Can you work these out from the model? Positions are in its coordinate system, mm. Give positions to 0.01 mm unless a question says otherwise; leave off trailing zeros. Order: outer loops, then holes, each group sorted by start corner. A loop starts at its lowest first (then second) coordinate and runs counter-clockwise, first axis right, second up. Notation, with made-up numbers: (26.5, 19) - (84.5, 19) arc R24 cw to (84.5, 31) - close; hole circle Ø9 at (12, 32.25). An arc over 180 degrees is marked (long way). Answer as a JSON object with one key per item and string values.
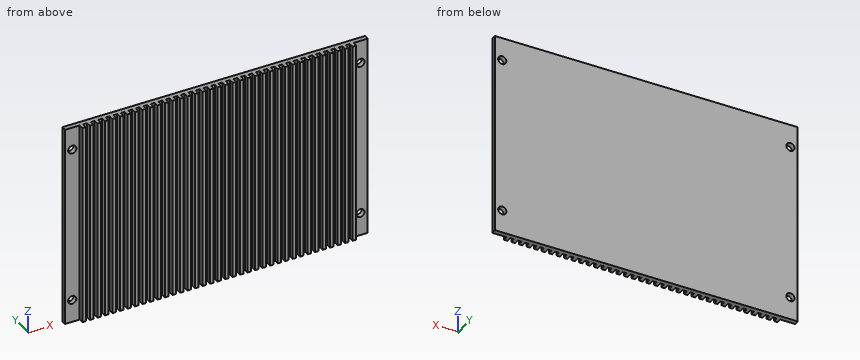
```python
from build123d import *

# Parameters (mm, degrees)
SKETCH1_W               = 125
SKETCH1_H               = 84
BOSS_EXTRUDE1_DEPTH     = 2
M3_CLEARANCE_HOLE1_D    = 3.4
MIRROR2_COPY_1_D        = 3.4
SKETCH4_W               = 1.5
SKETCH4_H               = 84
BOSS_EXTRUDE2_DEPTH     = 2
FILL_START              = -42
FILL_PATTERN2_OUTLINE_W = 1.5
FILL_PATTERN2_OUTLINE_H = 2
FILL_PATTERN2_DEPTH     = 84


# Read off the part's stored shape, not the designer's step: Fill Pattern2
with BuildPart() as part:
    # Sketch1 → Boss-Extrude1 (new body)
    with BuildSketch(Plane(origin=(0, 0, 0), x_dir=(1, 0, 0), z_dir=(0, 1, 0))):
        Rectangle(SKETCH1_W, SKETCH1_H)
    extrude(amount=BOSS_EXTRUDE1_DEPTH)

    # M3 Clearance Hole1 (through all)
    with Locations(Plane(origin=(0, 2, 0), x_dir=(1, 0, 0), z_dir=(0, 1, 0))):
        with Locations((-59.5, 32.5)):
            m3_clearance_hole1 = Hole(M3_CLEARANCE_HOLE1_D / 2)

    # Mirror1: M3 Clearance Hole1 across plane
    add(m3_clearance_hole1.mirror(Plane(origin=(0, 0, 0), x_dir=(0, 0, 1), z_dir=(1, 0, 0))), mode=Mode.SUBTRACT)

    # Mirror2: M3 Clearance Hole1 across plane
    add(m3_clearance_hole1.mirror(Plane.XY), mode=Mode.SUBTRACT)

    # Mirror2 copy 1 (through all)
    with Locations(Plane(origin=(0, 2, 0), x_dir=(-1, 0, 0), z_dir=(0, 1, 0))):
        with Locations((-59.5, 32.5)):
            Hole(MIRROR2_COPY_1_D / 2)

    # Sketch4 → Boss-Extrude2 (add)
    with BuildSketch(Plane(origin=(0, 0, 0), x_dir=(1, 0, 0), z_dir=(0, 1, 0))):
        with Locations((-55.7, 0)):
            Rectangle(SKETCH4_W, SKETCH4_H)
    extrude(amount=-BOSS_EXTRUDE2_DEPTH)

    # Fill Pattern2 outline → Fill Pattern2 (add)
    with BuildSketch(Plane.XY.offset(FILL_START)):
        with Locations((55.9, -1)):
            Rectangle(FILL_PATTERN2_OUTLINE_W, FILL_PATTERN2_OUTLINE_H)
        with Locations((52.8, -1)):
            Rectangle(FILL_PATTERN2_OUTLINE_W, FILL_PATTERN2_OUTLINE_H)
        with Locations((49.7, -1)):
            Rectangle(FILL_PATTERN2_OUTLINE_W, FILL_PATTERN2_OUTLINE_H)
        with Locations((46.6, -1)):
            Rectangle(FILL_PATTERN2_OUTLINE_W, FILL_PATTERN2_OUTLINE_H)
        with Locations((43.5, -1)):
            Rectangle(FILL_PATTERN2_OUTLINE_W, FILL_PATTERN2_OUTLINE_H)
        with Locations((40.4, -1)):
            Rectangle(FILL_PATTERN2_OUTLINE_W, FILL_PATTERN2_OUTLINE_H)
        with Locations((37.3, -1)):
            Rectangle(FILL_PATTERN2_OUTLINE_W, FILL_PATTERN2_OUTLINE_H)
        with Locations((34.2, -1)):
            Rectangle(FILL_PATTERN2_OUTLINE_W, FILL_PATTERN2_OUTLINE_H)
        with Locations((31.1, -1)):
            Rectangle(FILL_PATTERN2_OUTLINE_W, FILL_PATTERN2_OUTLINE_H)
        with Locations((28, -1)):
            Rectangle(FILL_PATTERN2_OUTLINE_W, FILL_PATTERN2_OUTLINE_H)
        with Locations((24.9, -1)):
            Rectangle(FILL_PATTERN2_OUTLINE_W, FILL_PATTERN2_OUTLINE_H)
        with Locations((21.8, -1)):
            Rectangle(FILL_PATTERN2_OUTLINE_W, FILL_PATTERN2_OUTLINE_H)
        with Locations((18.7, -1)):
            Rectangle(FILL_PATTERN2_OUTLINE_W, FILL_PATTERN2_OUTLINE_H)
        with Locations((15.6, -1)):
            Rectangle(FILL_PATTERN2_OUTLINE_W, FILL_PATTERN2_OUTLINE_H)
        with Locations((12.5, -1)):
            Rectangle(FILL_PATTERN2_OUTLINE_W, FILL_PATTERN2_OUTLINE_H)
        with Locations((9.4, -1)):
            Rectangle(FILL_PATTERN2_OUTLINE_W, FILL_PATTERN2_OUTLINE_H)
        with Locations((6.3, -1)):
            Rectangle(FILL_PATTERN2_OUTLINE_W, FILL_PATTERN2_OUTLINE_H)
        with Locations((3.2, -1)):
            Rectangle(FILL_PATTERN2_OUTLINE_W, FILL_PATTERN2_OUTLINE_H)
        with Locations((0.1, -1)):
            Rectangle(FILL_PATTERN2_OUTLINE_W, FILL_PATTERN2_OUTLINE_H)
        with Locations((-3, -1)):
            Rectangle(FILL_PATTERN2_OUTLINE_W, FILL_PATTERN2_OUTLINE_H)
        with Locations((-6.1, -1)):
            Rectangle(FILL_PATTERN2_OUTLINE_W, FILL_PATTERN2_OUTLINE_H)
        with Locations((-9.2, -1)):
            Rectangle(FILL_PATTERN2_OUTLINE_W, FILL_PATTERN2_OUTLINE_H)
        with Locations((-12.3, -1)):
            Rectangle(FILL_PATTERN2_OUTLINE_W, FILL_PATTERN2_OUTLINE_H)
        with Locations((-15.4, -1)):
            Rectangle(FILL_PATTERN2_OUTLINE_W, FILL_PATTERN2_OUTLINE_H)
        with Locations((-18.5, -1)):
            Rectangle(FILL_PATTERN2_OUTLINE_W, FILL_PATTERN2_OUTLINE_H)
        with Locations((-21.6, -1)):
            Rectangle(FILL_PATTERN2_OUTLINE_W, FILL_PATTERN2_OUTLINE_H)
        with Locations((-24.7, -1)):
            Rectangle(FILL_PATTERN2_OUTLINE_W, FILL_PATTERN2_OUTLINE_H)
        with Locations((-27.8, -1)):
            Rectangle(FILL_PATTERN2_OUTLINE_W, FILL_PATTERN2_OUTLINE_H)
        with Locations((-30.9, -1)):
            Rectangle(FILL_PATTERN2_OUTLINE_W, FILL_PATTERN2_OUTLINE_H)
        with Locations((-34, -1)):
            Rectangle(FILL_PATTERN2_OUTLINE_W, FILL_PATTERN2_OUTLINE_H)
        with Locations((-37.1, -1)):
            Rectangle(FILL_PATTERN2_OUTLINE_W, FILL_PATTERN2_OUTLINE_H)
        with Locations((-40.2, -1)):
            Rectangle(FILL_PATTERN2_OUTLINE_W, FILL_PATTERN2_OUTLINE_H)
        with Locations((-43.3, -1)):
            Rectangle(FILL_PATTERN2_OUTLINE_W, FILL_PATTERN2_OUTLINE_H)
        with Locations((-46.4, -1)):
            Rectangle(FILL_PATTERN2_OUTLINE_W, FILL_PATTERN2_OUTLINE_H)
        with Locations((-49.5, -1)):
            Rectangle(FILL_PATTERN2_OUTLINE_W, FILL_PATTERN2_OUTLINE_H)
        with Locations((-52.6, -1)):
            Rectangle(FILL_PATTERN2_OUTLINE_W, FILL_PATTERN2_OUTLINE_H)
    extrude(amount=FILL_PATTERN2_DEPTH)


solid = part.part
```
Q1. If we section it at A-A, the plane x = 59.5: Please give me the cut outline in (y, z), then the cut area to 3 significant figures.
Recorded:
{"outline": "(0, -42) - (2, -42) - (2, -34.2) - (0, -34.2) - close; (0, -30.8) - (2, -30.8) - (2, 30.8) - (0, 30.8) - close; (0, 34.2) - (2, 34.2) - (2, 42) - (0, 42) - close", "area": "154 mm^2"}
Q2. I'm going to push flat-ended pins straight in: pin 1 Ø0.6 at (y, z) = (-1.5, -14) entering from +X; pin 2 Ø1 at (y, z) = (-1, 13) entering from -X; pin 3 Ø0.8 at (x, z) = (-26, -9.5) entering from -Y. Where does each tip first touch, or does it pass through?
Recorded:
{"pin 1": "stops at x = 56.65", "pin 2": "stops at x = -56.45", "pin 3": "stops at y = 0"}
Q3. If we section it at B-B, the plane z = -32.5: Count the separate pieces of the cut face and the enclosed holes in it, then the cut area to 3 significant figures.
Recorded:
{"separate pieces": "3", "enclosed holes": "0", "area": "347 mm^2"}
Q4. I need wall thicknesses on L1, parallel to Z at x = -59.5, y = 1.1; L2, parallel to Y at x = 48.5, z = 26; L3, parallel to X at y = 0.55, z = 33.5. Which ranges of each line are inside material? Lowest first, please.
Recorded:
{"L1": "z = -42 to -34.2, -30.8 to 30.8, 34.2 to 42", "L2": "y = 0 to 2", "L3": "x = -62.5 to -60.87, -58.13 to 58.13, 60.87 to 62.5"}
